The listing builds one solid part. Answer for the finished solid, in the listing's coordinates (mm). Face numbers are marked on the shaded views. A direction names the side the tool comes from. Give positions to 0.01 mm unless a question says otherwise; leave off trailing zeros. Write each loop counter-clockwise with the first axis right and the second up, starting at its lowest first coordinate (ties: lowest second). Pieces come first, ordered by that corner, then holes.
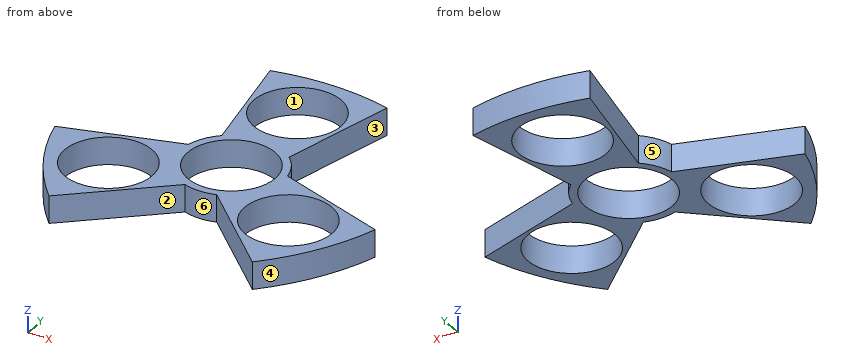
```python
from build123d import *

# Parameters (mm, degrees)
F0_R     = 11.2
F1_DEPTH = 7


with BuildPart() as f1:
    # F0 (on Top) → F1 (new body)
    with BuildSketch(Plane.XY):
        with BuildLine():
            ThreePointArc((4.141857, -12.533356), (10.698423, -7.731995), (13.2, 0))
            ThreePointArc((13.2, 0), (13.131104, 1.346893), (12.925133, 2.679725))
            ThreePointArc((12.925133, 2.679725), (11.431535, 6.6), (8.783277, 9.853631))
            ThreePointArc((8.783277, 9.853631), (0, 13.2), (-8.783277, 9.853631))
            ThreePointArc((-8.783277, 9.853631), (-11.431535, 6.6), (-12.925133, 2.679725))
            ThreePointArc((-12.925133, 2.679725), (-11.431535, -6.6), (-4.141857, -12.533356))
            ThreePointArc((-4.141857, -12.533356), (0, -13.2), (4.141857, -12.533356))
        make_face()
        Circle(F0_R, mode=Mode.SUBTRACT)
        with BuildLine():
            ThreePointArc((12.925133, 2.679725), (13.131104, 1.346893), (13.2, 0))
            ThreePointArc((13.2, 0), (10.698423, -7.731995), (4.141857, -12.533356))
            Line((4.141857, -12.533356), (26.512645, -33.127057))
            ThreePointArc((26.512645, -33.127057), (35.773086, -20.883133), (41.746416, -6.741393))
            Line((41.746416, -6.741393), (12.925133, 2.679725))
        make_face()
        with Locations((23.451635, -13.539808)):
            Circle(F0_R, mode=Mode.SUBTRACT)
        with BuildLine():
            ThreePointArc((-8.783277, 9.853631), (0, 13.2), (8.783277, 9.853631))
            Line((8.783277, 9.853631), (15.432551, 39.524153))
            ThreePointArc((15.432551, 39.524153), (0.19878, 41.421968), (-15.03499, 39.524153))
            Line((-15.03499, 39.524153), (-8.783277, 9.853631))
        make_face()
        with Locations((0, 27.079616)):
            Circle(F0_R, mode=Mode.SUBTRACT)
        with BuildLine():
            Line((-26.711425, -32.78276), (-4.141857, -12.533356))
            ThreePointArc((-4.141857, -12.533356), (-11.431535, -6.6), (-12.925133, 2.679725))
            Line((-12.925133, 2.679725), (-41.945196, -6.397096))
            ThreePointArc((-41.945196, -6.397096), (-35.971866, -20.538835), (-26.711425, -32.78276))
        make_face()
        with Locations((-23.451635, -13.539808)):
            Circle(F0_R, mode=Mode.SUBTRACT)
    extrude(amount=F1_DEPTH)


solid = f1.part
```
Item 1: Consider probe 1 along Y at (x, z) = (0, 5); probe 2 along Y at (x, z) = (3, 3.75); probe 3 along X at (y, z) = (7.5, 3). Determine where each line is inside the solid, lowest interval first.
Conclusion:
probe 1: y = -13.2 to -11.2, 11.2 to 15.88, 38.28 to 41.42
probe 2: y = -12.85 to -10.79, 10.79 to 16.29, 37.87 to 41.36
probe 3: x = -10.86 to -8.32, 8.32 to 10.86
Item 2: Which of the six approach directions +Z, -Z, +X, -X, +Y, -Y give full straight-line access (tool end or side, diameter ignored) to the marked faces 1, 2 and 3?
Conclusion:
face 1: +Z, -Z
face 2: +Z, -Z, -Y
face 3: +Z, -Z, +X
Item 3: A cutting plane is placed at A-A, the plane x = 19.5. Give the vertices of the cut face in (y, z), plus the area to 3 significant figures.
Conclusion:
outline: (-26.67, 0) - (-24.02, 0) - (-24.02, 7) - (-26.67, 7) - close; (-3.06, 0) - (0.53, 0) - (0.53, 7) - (-3.06, 7) - close
area: 43.7 mm2
Item 4: A cutting plane is placed at B-B, the plane y = -26.5. Give the vertices of the cut face in (x, z).
Conclusion:
outline: (-32.06, 0) - (-19.71, 0) - (-19.71, 7) - (-32.06, 7) - close; (19.31, 0) - (32.11, 0) - (32.11, 7) - (19.31, 7) - close
Item 5: A cutting plane is placed at C-C, the plane z = 5. Give the vertices of the cut face in (x, y) (3 decimals).
Conclusion:
outline: (-41.945, -6.397) arc R62.09 ccw to (-26.711, -32.783) - (-4.142, -12.533) arc R13.2 ccw to (4.142, -12.533) - (26.513, -33.127) arc R62.09 ccw to (41.746, -6.741) - (12.925, 2.68) arc R13.2 ccw to (8.783, 9.854) - (15.433, 39.524) arc R62.09 ccw to (-15.035, 39.524) - (-8.783, 9.854) arc R13.2 ccw to (-12.925, 2.68) - close; hole circle Ø22.4 at (-23.452, -13.54); hole circle Ø22.4 at (0, 0); hole circle Ø22.4 at (0, 27.08); hole circle Ø22.4 at (23.452, -13.54)
Item 6: A cutting plane is placed at D-D, the plane x = 0. Give the vertices of the cut face in (y, z), plus the area to 3 significant figures.
Conclusion:
outline: (-13.2, 0) - (-11.2, 0) - (-11.2, 7) - (-13.2, 7) - close; (11.2, 0) - (15.88, 0) - (15.88, 7) - (11.2, 7) - close; (38.28, 0) - (41.42, 0) - (41.42, 7) - (38.28, 7) - close
area: 68.8 mm2
Item 7: Each of these flat-tipped pins is pushed along its axis until it touches: P1, Ø4, axis at x = 9.5, z = 5, coming from the +Y side; P2, Ø8, axis at x = 12.5, y = 32, coming from the -Z side; P3, Ø1.5, axis at y = -8.5, z = 3, coming from the -X side; P4, Ø13.5, axis at x = 23.45, y = -13.54, coming from the +Z side. Where does it stop, or does it pass through?
Conclusion:
P1: stops at y = 40.99
P2: stops at z = 0
P3: stops at x = -41.55
P4: passes through
Item 8: Determine the mould class of the marked faces 4, 5 and 6 for opening direction X: pulls with the +X half, pulls with the -X half, needs draft (parallel to the pull), parting line crosses it, or undercut.
Conclusion:
face 4: pulls with the +X half
face 5: pulls with the -X half
face 6: undercut
